```python
from build123d import *

# Parameters (mm, degrees)
SKETCH_1_W          = 45
SKETCH_1_H          = 45
EXTRUDE_1_DEPTH     = 10
SKETCH_2_R          = 4
CUT_EXTRUDE_4_DEPTH = 34.35416016
SKETCH_3_R          = 15
CUT_EXTRUDE_5_DEPTH = 4
SKETCH_4_R          = 8
CUT_EXTRUDE_6_DEPTH = 4
SKETCH_5_R          = 1.5
CUT_EXTRUDE_7_DEPTH = 34.35416016
CUT_EXTRUDE_8_DEPTH = 5
CHAMFER_1_SIZE      = 1
SKETCH_7_R          = 6
CUT_EXTRUDE_9_DEPTH = 33.810059433


with BuildPart() as part:
    # 草图1 → 凸台-拉伸1 (new body)
    with BuildSketch(Plane(origin=(0, 0, 0), x_dir=(1, 0, 0), z_dir=(0, 1, 0))):
        Rectangle(SKETCH_1_W, SKETCH_1_H)
    extrude(amount=EXTRUDE_1_DEPTH)

    # 草图2 → 切除-拉伸4 (cut, through all)
    with BuildSketch(Plane(origin=(0, 0, 0), x_dir=(1, 0, 0), z_dir=(0, 1, 0))):
        with Locations(Location((0, 3, 0), (0, 0, 270))):
            Circle(SKETCH_2_R)
    extrude(amount=CUT_EXTRUDE_4_DEPTH, mode=Mode.SUBTRACT)

    # 草图3 → 切除-拉伸5 (cut)
    with BuildSketch(Plane.XZ):
        with Locations(Location((0, -3, 0), (0, 0, 270))):
            Circle(SKETCH_3_R)
    extrude(amount=-CUT_EXTRUDE_5_DEPTH, mode=Mode.SUBTRACT)

    # 草图4 → 切除-拉伸6 (cut)
    with BuildSketch(Plane.XZ.offset(-4)):
        with Locations(Location((0, -3, 0), (0, 0, 270))):
            Circle(SKETCH_4_R)
    extrude(amount=-CUT_EXTRUDE_6_DEPTH, mode=Mode.SUBTRACT)

    # 草图5 → 切除-拉伸7 (cut, through all)
    with BuildSketch(Plane(origin=(0, 10, 0), x_dir=(1, 0, 0), z_dir=(0, 1, 0))):
        with Locations(Location((-19.5, 19.5, 0), (0, 0, 270))):
            Circle(SKETCH_5_R)
        with Locations(Location((19.5, 19.5, 0), (0, 0, 90))):
            Circle(SKETCH_5_R)
        with Locations(Location((19.5, -19.5, 0), (0, 0, 270))):
            Circle(SKETCH_5_R)
        with Locations(Location((-19.5, -19.5, 0), (0, 0, 90))):
            Circle(SKETCH_5_R)
    extrude(amount=-CUT_EXTRUDE_7_DEPTH, mode=Mode.SUBTRACT)

    # 草图6 → 切除-拉伸8 (cut)
    with BuildSketch(Plane(origin=(0, 10, 0), x_dir=(1, 0, 0), z_dir=(0, 1, 0))):
        with BuildLine():
            Line((-16.5, 22.5), (-16.5, 19.5))
            ThreePointArc((-16.5, 19.5), (-17.378679656, 17.378679656), (-19.5, 16.5))
            Line((-19.5, 16.5), (-22.5, 16.5))
            Line((-22.5, 16.5), (-22.5, 22.5))
            Line((-22.5, 22.5), (-16.5, 22.5))
        make_face()
        with BuildLine():
            Line((22.5, 16.5), (22.5, 22.5))
            Line((22.5, 22.5), (16.5, 22.5))
            Line((16.5, 22.5), (16.5, 19.5))
            ThreePointArc((16.5, 19.5), (17.378679656, 17.378679656), (19.5, 16.5))
            Line((19.5, 16.5), (22.5, 16.5))
        make_face()
        with BuildLine():
            Line((19.5, -16.5), (22.5, -16.5))
            Line((22.5, -16.5), (22.5, -22.5))
            Line((22.5, -22.5), (16.5, -22.5))
            Line((16.5, -22.5), (16.5, -19.5))
            ThreePointArc((16.5, -19.5), (17.378679656, -17.378679656), (19.5, -16.5))
        make_face()
        with BuildLine():
            Line((-22.5, -16.5), (-22.5, -22.5))
            Line((-22.5, -22.5), (-16.5, -22.5))
            Line((-16.5, -22.5), (-16.5, -19.5))
            ThreePointArc((-16.5, -19.5), (-17.378679656, -17.378679656), (-19.5, -16.5))
            Line((-19.5, -16.5), (-22.5, -16.5))
        make_face()
    extrude(amount=-CUT_EXTRUDE_8_DEPTH, mode=Mode.SUBTRACT)

    # 倒角1
    chamfer_1_edges = [part.edges().sort_by_distance(p)[0] for p in [
        (22.5, 2.5, 22.5),
        (-22.5, 2.5, 22.5),
        (-22.5, 2.5, -22.5),
        (22.5, 2.5, -22.5),
    ]]
    chamfer(chamfer_1_edges, length=CHAMFER_1_SIZE)

    # 草图7 → 切除-拉伸9 (cut, through all)
    with BuildSketch(Plane.XZ.offset(-8)):
        with Locations(Location((0, -3, 0), (0, 0, 270))):
            Circle(SKETCH_7_R)
    extrude(amount=-CUT_EXTRUDE_9_DEPTH, mode=Mode.SUBTRACT)


solid = part.part
```
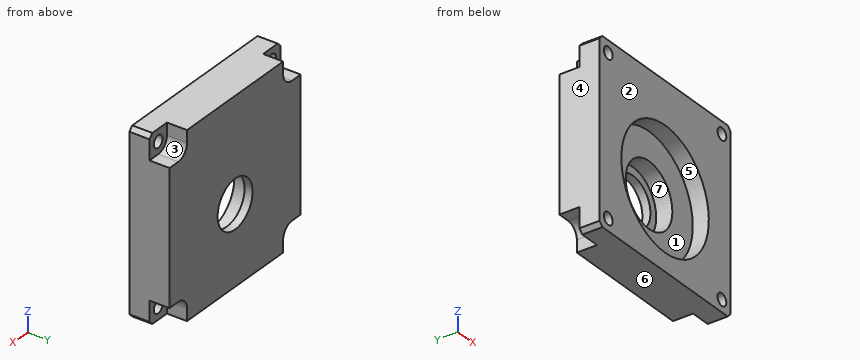
Can you work these out from the model? Positions are in its coordinate system, mm. Face numbers are marked on the shaded views. A direction names the side the tool comes from. Round coordinates to 2 decimals unless told otherwise and drop trailing zeros. Loops run counter-clockwise (first coordinate to the right, second up) from the corner with the lowest first, then second, coordinate; pieces in that order, holes last.
Item 1: Will these pins go through, and if not, where does the flat tip stop? pin 1 Ø0.9 at (y, z) = (7, -21) entering from -X; pin 2 Ø2.5 at (y, z) = (7.5, 21) entering from +X; pin 3 Ø1.8 at (x, z) = (20, -20.5) entering from +Y.
Item 2: Please list where these lines run through material, in increasing order: L1, parallel to X at y = 1.25, z = 19.5; L2, parallel to Z at x = -20, y = 3.25; L3, parallel to X at y = 9.55, z = -3.
Item 3: Suppose I cut it at A-A, the plane z = -3. Write out the boundary of the cut face in (x, y), then the cut area to 3 significant figures.
Item 4: If we mould it in two halves opening along Z, with no side actions, what happens to the marked faces 4, 5, 6 and 7? For each: +Z half, -Z half, draft (parallel to the pull), parting line (faces both ways), or undercut.
Item 5: Suppose I cut it at B-B, the plane y = 1.5. Write out the boundary of the cut face in (x, z).
Item 6: Suppose I cut it at D-D, the plane x = 7. Write out the boundary of the cut face in (y, z), then the cut area to 3 significant figures.
Item 7: Suppose I cut it at C-C, the plane x = 2.5. Write out the boundary of the cut face in (y, z).
Item 8: Which directions (+Z, -Z, +X, -X, +Y, -Y) give clear straight access to the entire face, cutting with the end or side of a thin tool? Please do the marked faces 1, 2 and 3.
Reported:
1. pin 1: stops at x = -16.5
1. pin 2: stops at x = 16.5
1. pin 3: stops at y = 5
2. L1: x = -22.5 to -21, -18 to 18, 21 to 22.5
2. L2: z = -22.5 to -20.91, -18.09 to 18.09, 20.91 to 22.5
2. L3: x = -22.5 to -6, 6 to 22.5
3. outline: (-22.5, 0) - (-15, 0) - (-15, 4) - (-8, 4) - (-8, 8) - (-6, 8) - (-6, 10) - (-22.5, 10) - close; (6, 8) - (8, 8) - (8, 4) - (15, 4) - (15, 0) - (22.5, 0) - (22.5, 10) - (6, 10) - close
3. area: 242 mm2
4. face 4: draft
4. face 5: undercut
4. face 6: -Z half
4. face 7: undercut
5. outline: (-22.5, -21.5) - (-21.5, -22.5) - (21.5, -22.5) - (22.5, -21.5) - (22.5, 21.5) - (21.5, 22.5) - (-21.5, 22.5) - (-22.5, 21.5) - close; hole circle Ø3 at (-19.5, -19.5); hole circle Ø3 at (-19.5, 19.5); hole circle Ø30 at (0, -3); hole circle Ø3 at (19.5, -19.5); hole circle Ø3 at (19.5, 19.5)
6. outline: (0, -22.5) - (10, -22.5) - (10, 22.5) - (0, 22.5) - (0, 10.27) - (4, 10.27) - (4, 0.87) - (8, 0.87) - (8, -6.87) - (4, -6.87) - (4, -16.27) - (0, -16.27) - close
6. area: 313 mm2
7. outline: (0, -22.5) - (10, -22.5) - (10, -8.45) - (8, -8.45) - (8, -10.6) - (4, -10.6) - (4, -17.79) - (0, -17.79) - close; (0, 11.79) - (4, 11.79) - (4, 4.6) - (8, 4.6) - (8, 2.45) - (10, 2.45) - (10, 22.5) - (0, 22.5) - close
8. face 1: -Y
8. face 2: +Z, -Z, +X, -X, -Y
8. face 3: +Z, +X, +Y
